from build123d import *

# Parameters (mm, degrees)
F0_R          = 4.7625
F0_R_2        = 3.175
F3_DEPTH      = 25.4
F3_DEPTH_BACK = 25.4


with BuildPart() as f2:
    # F1 (on Front) → F2 (revolve)
    with BuildSketch(Plane.XZ):
        with BuildLine():
            Line((-50.8, 0), (0, 0))
            Line((0, 0), (46.0375, 0))
            ThreePointArc((46.0375, 0), (43.7126600757, 5.6126600757), (38.1, 7.9375))
            ThreePointArc((38.1, 7.9375), (33.6653909537, 6.5831716411), (30.7440837762, 2.9823485307))
            Line((30.7440837762, 2.9823485307), (10.4464940581, 3.7892503407))
            ThreePointArc((10.4464940581, 3.7892503407), (0.4414129771, 11.1037295912), (-10.1127308342, 4.6065530849))
            Line((-10.1127308342, 4.6065530849), (-26.5403060608, 5.2596079731))
            ThreePointArc((-26.5403060608, 5.2596079731), (-40.7909001256, 12.4116500319), (-50.8, 0))
        make_face()
    revolve(axis=Axis((-25.4, 0, 0), (-1, 0, 0)))

    # F0 (on Top) → F3 (cut, two sides)
    with BuildSketch(Plane.XY) as f3_sk:
        Circle(F0_R)
        with Locations((38.1, 0)):
            Circle(F0_R_2)
    extrude(amount=-F3_DEPTH, mode=Mode.SUBTRACT)
    extrude(f3_sk.sketch, amount=F3_DEPTH_BACK, mode=Mode.SUBTRACT)

    # F4 (on Front) → F5 (revolve)
    with BuildSketch(Plane.XZ):
        with BuildLine():
            Line((38.1, 57.15), (38.1, 0))
            Line((38.1, 0), (38.1, -8.0190747976))
            Line((38.1, -8.0190747976), (41.275, -8.0190747976))
            Line((41.275, -8.0190747976), (41.275, 7.316250355))
            Line((41.275, 7.316250355), (42.6851746338, 7.316250355))
            Line((42.6851746338, 7.316250355), (42.8192897481, 9.1268108057))
            add(Edge.make_bspline(
                [(38.1, 57.15), (38.6338089941, 57.2602124833), (39.9620793922, 57.5351315702), (43.3864941638, 54.4836217076), (45.3763277656, 50.0233180211), (39.8347693404, 11.9671706067), (42.1115041372, 9.4275469633), (42.6981474798, 9.1602681559), (42.8192897481, 9.1268108057)],
                knots=[0, 0, 0, 0, 0.0915460023, 0.2276474816, 0.3916091393, 0.8222909766, 0.937828958, 0.9674329102, 0.9674329102, 0.9674329102, 0.9674329102], degree=3))
        make_face()
    revolve(axis=Axis((38.1, 0, 28.575), (0, 0, 1)))


solid = f2.part
CAD build for the part. Positions are in the model's coordinates, mm. A direction names the side the tool comes from. Give positions to 0.01 mm unless a question says otherwise; leave off trailing zeros. Loops run counter-clockwise (first coordinate to the right, second up) from the corner with the lowest first, then second, coordinate; pieces in that order, holes last. Notation, with made-up numbers: M 42.5,-29.75 L 64.5,-29.75 A26 ccw 64.5,0.25 Z; hole C 44.5,8.25 d9. An arc over 180 degrees is marked long. Write each question's results on one line, items separated by ' | '.
Q1. Probe probe 1 along X at (y, z) = (0, -7.25); probe 2 along X at (y, z) = (0, -7.5) (1 decimal); probe 3 along X at (y, z) = (0, 4.25). List the from-to ranges inside material, lowest first.
Geometry check:
probe 1: x = -48.53 to -27.67, -8.42 to -4.76, 4.76 to 8.42, 34.87 to 41.33 | probe 2: x = -48.3 to -27.9, -8.2 to -4.8, 4.8 to 8.2, 34.9 to 41.3 | probe 3: x = -50.07 to -4.76, 4.76 to 10.27, 31.4 to 44.8
Q2. Band-saw the part on A-A on x = -1.5. Write the cut outline in (y, z).
Geometry check:
outline: M -4.52,-10.04 L -4.52,10.04 A11.01 ccw Z; M 4.52,-10.04 A11.01 ccw 4.52,10.04 Z
Q3. Flat gauge pins, fed straight in: P1, Ø8, axis at x = -11, z = 0.5, coming from the -Y side; P2, Ø3, axis at x = 39.5, y = 1.5, coming from the -Z side; P3, Ø1.5, axis at x = 2.5, y = 3.5, coming from the -Z side; P4, Ø8.5, axis at x = 0, y = 0, coming from the -Z side. Where does each tip first touch, or does it go through?
Geometry check:
P1: stops at y = -8.62 | P2: stops at z = -8.02 | P3: stops at z = -10.04 | P4: passes through
Q4. Which spindle directions (+Z, -Z, +X, -X, +Y, -Y) get a long thin tool onto all of the face, cutting with end or side? Do faces 1 (the face through (-18.44, -4.82, -1.07)), 2 (the face through (35.58, -1.93, -7.64)). Say none if no direction does.
Geometry check:
face 1: none | face 2: -Z
Q5. Band-saw the part on B-B on x = -19.5. Write the cut outline in (y, z), and give its area (3 significant figures).
Geometry check:
outline: C 0,0 d9.96 | area: 77.9 mm²
Q6. Mould opens along X. For faces 3 (the face through (42.37, -1.77, 7.83)), 4 (the face through (38, 0, -8.019)) say: pulls with the +X half, pulls with the -X half, needs draft (parallel to the pull), parting line crosses it, or undercut.
Geometry check:
face 3: undercut | face 4: needs draft
Q7. Band-saw the part on C-C on x = 27. Write the cut outline in (y, z).
Geometry check:
outline: C 0,0 d6.26
